from build123d import *

# Parameters (mm, degrees)
F0_W           = 65
F0_H           = 29.5
F0_R           = 6.35
F1_DEPTH       = 25
F2_SIZE        = 0.5
F3_R           = 6.35
F4_DEPTH       = 8
F5_SIZE        = 2
F7_D           = 3.2
F7_DEPTH       = 8
F7_TIP         = 0.9613769904
F9_D           = 3.3
F9_CBORE_D     = 6.5
F9_CBORE_DEPTH = 3
F11_D          = 3.2
F11_DEPTH      = 10
F11_TIP        = 0.9613769904


with BuildPart() as f1:
    # F0 (on Front) → F1 (new body)
    with BuildSketch(Plane.XZ):
        with Locations((0, 3.25)):
            Rectangle(F0_W, F0_H)
        Circle(F0_R, mode=Mode.SUBTRACT)
    extrude(amount=F1_DEPTH)

    # F2
    f2_edges = [f1.edges().sort_by_distance(p)[0] for p in [
        (-32.5, -12.5, 18),
        (32.5, -12.5, 18),
    ]]
    chamfer(f2_edges, length=F2_SIZE)

    # F3 (on face) → F4 (cut)
    with BuildSketch(Plane.XZ.offset(25)):
        with BuildLine():
            ThreePointArc((6.0621778265, -11.5), (11.1312243654, -6.7153439322), (13, 0))
            ThreePointArc((13, 0), (-6.7153439322, 11.1312243654), (-6.0621778265, -11.5))
            Line((-6.0621778265, -11.5), (6.0621778265, -11.5))
        make_face()
        Circle(F3_R, mode=Mode.SUBTRACT)
    extrude(amount=-F4_DEPTH, mode=Mode.SUBTRACT)

    # F5
    f5_edges = [f1.edges().sort_by_distance(p)[0] for p in [
        (32.5, -12.5, -11.5),
        (-32.5, -12.5, -11.5),
    ]]
    chamfer(f5_edges, length=F5_SIZE)

    # F7
    with Locations(Plane.XY.offset(18)):
        with Locations((12.5, -6.25), (12.5, -18.75), (-12.5, -6.25), (-12.5, -18.75)):
            Hole(F7_D / 2, depth=F7_DEPTH)
            with Locations((0, 0, -(F7_DEPTH + F7_TIP / 2))):  # 118° drill point
                Cone(0, F7_D / 2, F7_TIP, mode=Mode.SUBTRACT)

    # F9 (through all)
    with Locations(Plane.XY.offset(18)):
        with Locations((-25, -8.5), (-25, -16.5), (25, -8.5), (25, -16.5)):
            CounterBoreHole(F9_D / 2, F9_CBORE_D / 2, F9_CBORE_DEPTH)

    # F11
    with Locations(Plane.XZ.offset(17)):
        with Locations((0, 9.53), (8.2532220981, -4.765), (-8.2532220981, -4.765)):
            Hole(F11_D / 2, depth=F11_DEPTH)
            with Locations((0, 0, -(F11_DEPTH + F11_TIP / 2))):  # 118° drill point
                Cone(0, F11_D / 2, F11_TIP, mode=Mode.SUBTRACT)


solid = f1.part
Model file for the job. Use its own axes, mm. A direction names the side the tool comes from. Give positions to 0.01 mm unless a question says otherwise; leave off trailing zeros. Loops run counter-clockwise (first coordinate to the right, second up) from the corner with the lowest first, then second, coordinate; pieces in that order, holes last.
1) Saw through at C-C (y = -4). Write the cut outline in (x, z), plus the area to 3 significant figures.
2) Flat gauge pins, fed straight in: pin 1 Ø14.5 at (x, z) = (0, 0) entering from -Y; pin 2 Ø2.5 at (x, y) = (12.5, -18.75) entering from +Z; pin 3 Ø3 at (x, y) = (-25.5, -7.5) entering from +Z. Where does each tip first touch, or does it go through?
3) Saw through at A-A (z = -2). Write the cut outline in (x, y), plus the area to 3 significant figures.
4) Saw through at B-B (x = 25). Write the cut outline in (y, z), plus the area to 3 significant figures.
5) Pull direction Z, two halves, no side cores. Call faces 4 (the cylindrical face through (-10.9, -6.2, 13.9)), 5 (the cylindrical face through (0.208, -11.93, 11.116)), 6 (the conical face through (-12.54, -18.47, 9.21)): +Z half, -Z half, draft (parallel to the pull), parting line (faces both ways), or undercut.
6) Tool access for faces 1 (the cylindrical face through (-11.32, -17.67, 13.94)), 2 (the flat face through (-3, -17, 6)), 3 (the flat face through (32.5, -12, 4)): list every direction of +Z, -Z, +X, -X, +Y, -Y with a clear straight run to the whole face (end or side of a thin tool).
7) Wall check: line 1 (Y direction, x = 25, z = 16); line 2 (Y direction, x = 25, z = 7); line 3 (X direction, y = -21, z = 0). Give the ranges that are in metal, low to high.
8) Saw through at D-D (z = -8). Write the cut outline in (x, y).
Answer block:
1. outline: (-32.5, -9.5) - (-30.5, -11.5) - (30.5, -11.5) - (32.5, -9.5) - (32.5, 17.5) - (32, 18) - (-32, 18) - (-32.5, 17.5) - close; hole circle Ø12.7 at (0, 0)
1. area: 1,790 mm2
2. pin 1: stops at y = -17
2. pin 2: stops at z = 9.79
2. pin 3: stops at z = 15
3. outline: (-32.5, -25) - (-12.85, -25) - (-12.85, -17) - (-6.03, -17) - (-6.03, 0) - (-32.5, 0) - close; (6.03, -17) - (12.85, -17) - (12.85, -25) - (32.5, -25) - (32.5, 0) - (6.03, 0) - close; hole circle Ø3.3 at (-25, -16.5); hole circle Ø3.3 at (-25, -8.5); hole circle Ø3.3 at (25, -16.5); hole circle Ø3.3 at (25, -8.5)
3. area: 1,180 mm2
4. outline: (-25, -11.5) - (-18.15, -11.5) - (-18.15, 15) - (-19.75, 15) - (-19.75, 18) - (-25, 18) - close; (-14.85, -11.5) - (-10.15, -11.5) - (-10.15, 15) - (-11.75, 15) - (-11.75, 18) - (-13.25, 18) - (-13.25, 15) - (-14.85, 15) - close; (-6.85, -11.5) - (0, -11.5) - (0, 18) - (-5.25, 18) - (-5.25, 15) - (-6.85, 15) - close
4. area: 524 mm2
5. face 4: draft
5. face 5: undercut
5. face 6: +Z half
6. face 1: +Z
6. face 2: -Y
6. face 3: +Z, -Z, +X, +Y, -Y
7. line 1: y = -25 to -19.75, -13.25 to -11.75, -5.25 to 0
7. line 2: y = -25 to -18.15, -14.85 to -10.15, -6.85 to 0
7. line 3: x = -32.5 to -13, 13 to 32.5
8. outline: (-32.5, -25) - (-10.25, -25) - (-10.25, -17) - (10.25, -17) - (10.25, -25) - (32.5, -25) - (32.5, 0) - (-32.5, 0) - close; hole circle Ø3.3 at (-25, -16.5); hole circle Ø3.3 at (-25, -8.5); hole circle Ø3.3 at (25, -16.5); hole circle Ø3.3 at (25, -8.5)
